Solid Edge part; units mm, degrees
sketch "Sketch1" plane through (0, 0, 0) normal (0, 0, 1) x (1, 0, 0)
  line L0 (-30, 75) -> (-30, -75)
  line L1 (-30, -75) -> (30, -75)
  line L2 (30, -75) -> (30, 75)
  line L3 (30, 75) -> (-30, 75)
extrude "Protrusion1" add sketch "Sketch1" along normal mid plane 30
sketch "Sketch2" plane through (0, 0, -15) normal (0, 0, -1) x (-1, 0, 0)
  circle A0 centre (0, 75) radius 30
extrude "ExtrudedCutout_1" cut sketch "Sketch2" against normal blind 30
sketch "Sketch3" plane through (0, 0, -15) normal (0, 0, -1) x (-1, 0, 0)
  circle A0 centre (0, 75) radius 30
  circle A1 centre (0, 75) radius 15
extrude "ExtrudedProtrusion_2" add sketch "Sketch3" against normal blind 40
sketch "Sketch4" plane through (0, 0, 15) normal (0, 0, 1) x (0, -1, 0)
  line L0 (75, 90) -> (75, 30)
  line L1 (75, 30) -> (25, 30)
  line L2 (25, 30) -> (25, 90)
  arc A0 (25, 90) -> (75, 90) centre (50, 90) cw
  circle A1 centre (50, 90) radius 10
  line L3 (75, -90) -> (75, -30)
  line L4 (75, -30) -> (25, -30)
  line L5 (25, -30) -> (25, -90)
  arc A2 (25, -90) -> (75, -90) centre (50, -90) ccw
  circle A3 centre (50, -90) radius 10
extrude "ExtrudedProtrusion_5" add sketch "Sketch4" against normal blind 30
sketch "Sketch5" plane through (0, 0, 0) normal (1, 0, 0) x (0, 1, 0)
  line L0 (-75, 15) -> (-59.5434, 94.7565)
  line L1 (5, 15) -> (-10.4566, 94.7565)
  line L2 (-75, 15) -> (5, 15)
  arc A0 (-59.5433, 94.7565) -> (-10.4567, 94.7565) centre (-35, 90) cw
  circle A1 centre (-35, 90) radius 12.5
extrude "ExtrudedProtrusion_6" add sketch "Sketch5" along normal mid plane 60
sketch "Sketch6" plane through (0, 0, 0) normal (1, 0, 0) x (0, 1, 0)
  line L0 (-75, 15) -> (-59.5434, 94.7565)
  line L1 (5, 15) -> (-10.4566, 94.7565)
  line L2 (-75, 15) -> (5, 15)
  arc A0 (-59.5433, 94.7565) -> (-10.4567, 94.7565) centre (-35, 90) cw
extrude "ExtrudedCutout_2" cut sketch "Sketch6" along normal mid plane 30
Could you check a few things on this model? Use its own coordinates, in mm. A direction names the side the tool comes from. Coordinates: 2 decimals unless noted, no trailing zeros. Loops run counter-clockwise (first coordinate to the right, second up) from the corner with the lowest first, then second, coordinate; pieces in that order, holes last. Notation, with made-up numbers: M -14,-28.5 L 15,-28.5 A14 ccw 15,-19.5 Z; hole C -11,65 d4. An arc over 180 degrees is marked long. Put each result on its own line as item: value. Start each with the question number.
(1) Suppose I cut it at B-B on x = 0. Please give me the cut outline in (y, z), then the cut area to 3 significant figures.
(2) I need wall thicknesses on line 1 (X direction, y = -50, z = 0.5); line 2 (X direction, y = -3, z = 31); line 3 (Y direction, x = 0, z = 2). Which ranges of each line are inside material? Lowest first, please. Write a range as from..to.
(3) Thinking about a two-plate mould opening in Y: for faces 1 (the face through (22, -35, 115)), 2 (the face through (-6, 89, 25)), 3 (the face through (0, 1, 15)), which applies, pulls with the +Y half, pulls with the -Y half, needs draft (parallel to the pull), parting line crosses it, or undercut?
(4) Suppose I cut it at C-C on z = 20.5. Please give me the cut outline in (x, y), then the cut area to 3 significant figures.
(5) Suppose I cut it at D-D on z = -2.5. Please give me the cut outline in (x, y), then the cut area to 3 significant figures.
(6) Will these pins go through, and if not, where does the flat tip stop? P1, Ø2, axis at x = -4, y = -18.5, coming from the +Z side; P2, Ø8, axis at y = -25, z = 44, coming from the +X side; P3, Ø1, axis at x = -18.5, y = -21.5, coming from the +Z side.
(7) Suppose I cut it at A-A on y = -35. Please give me the cut outline in (x, z).
(8) For faces 4 (the face through (-60, -25, 0)), 5 (the face through (3.905, 104.745, 9.164)), 6 (the face through (60, -25, 0)), which set-ups out of +Z, -Z, +X, -X, +Y, -Y let a thin tool reach every point of the face, with its end or its side?
Solutions:
1. outline: M -75,-15 L 60,-15 L 60,25 L 45,25 L 45,15 L -75,15 Z; M 90,-15 L 105,-15 L 105,25 L 90,25 Z
1. area: 4,800 mm2
2. line 1: x = -115..-100, -80..80, 100..115
2. line 2: x = -30..-15, 15..30
2. line 3: y = -75..60, 90..105
3. face 1: parting line crosses it
3. face 2: needs draft
3. face 3: undercut
4. outline: M -30,-73.93 L -15,-73.93 L -15,3.93 L -30,3.93 Z; C 0,75 d60; M 15,-73.93 L 30,-73.93 L 30,3.93 L 15,3.93 Z; hole C 0,75 d30
4. area: 4,460 mm2
5. outline: M -90,-75 L 90,-75 A25 ccw 90,-25 L 30,-25 L 30,75 A30 ccw -30,75 L -30,-25 L -90,-25 A25 ccw Z; hole C -90,-50 d20; hole C 0,75 d30; hole C 90,-50 d20
5. area: 17,000 mm2
6. P1: stops at z = 15
6. P2: stops at x = 30
6. P3: stops at z = 111.35
7. outline: M -110,-15 L 110,-15 L 110,15 L 30,15 L 30,77.5 L 15,77.5 L 15,15 L -15,15 L -15,77.5 L -30,77.5 L -30,15 L -110,15 Z; M -30,102.5 L -15,102.5 L -15,115 L -30,115 Z; M 15,102.5 L 30,102.5 L 30,115 L 15,115 Z
8. face 4: +Z, -Z, -X, +Y
8. face 5: +Z
8. face 6: +Z, -Z, +X, +Y
